Build history of the part. All positions in model axes, mm. A direction names the side the tool comes from. Round coordinates to 2 decimals unless told otherwise and drop trailing zeros. Order: outer loops, then holes, each group sorted by start corner. A loop starts at its lowest first (then second) coordinate and runs counter-clockwise, first axis right, second up. Notation, with made-up numbers: M 45,-6 L 70,-6 A13 ccw 70,7 Z; hole C -30.75,-6.5 d10. An arc over 180 degrees is marked long. Use CSV: the item, a comma, the result in double quotes.
Autodesk Inventor part; units mm, degrees
ref_plane "YZ Plane" through (0, 0, 0) normal (1, 0, 0) x (0, 1, 0)
ref_plane "XZ Plane" through (0, 0, 0) normal (0, 1, 0) x (-1, 0, 0)
ref_plane "XY Plane" through (0, 0, 0) normal (0, 0, 1) x (1, 0, 0)
sketch "Sketch1" plane through (0, 0, 0) normal (1, 0, 0) x (0, 1, 0)
  circle A0 centre (0, 0) radius 10
  circle A1 centre (0, 0) radius 20
  circle A2 centre (0, 0) radius 40
  circle A3 centre (0, 0) radius 50
  dimension "d0" = 20
  dimension "d1" = 40
  dimension "d2" = 80
  dimension "d3" = 100
extrude "Extrusion1" add sketch "Sketch1" along normal mid plane 40
extrude "Extrusion2" add sketch "Sketch1" along normal mid plane 30 contours A2
fillet "Fillet1" radius 2 1 edges at (-15, -40, 0)
fillet "Fillet4" radius 2 1 edges at (15, -40, 0)
fillet "Fillet5" radius 2 1 edges at (-15, -20, 0)
fillet "Fillet6" radius 2 1 edges at (15, -20, 0)
(1) Drop flat-ended pins along their axis: pin 1 (2 mm diameter, centred on y = 16.5, z = -15, fed in from -X); pin 2 (4 mm diameter, centred on y = -29.5, z = 23.5, fed in from +X); pin 3 (12 mm diameter, centred on x = 9, y = -35, fed in from -Z). Give the stop position or say it passes through.
Answer block:
pin 1,"stops at x = -15.13"
pin 2,"stops at x = 15.97"
pin 3,"stops at z = -40.73"
(2) Two-plate mould, pull along Y, no slides. Class faces 1 (the face through (18.479, -4.336, 19.524)), 2 (the face through (20, -5, 9)), 3 (the face through (-0.28, 47.69, -15.02)): released by +Y, released by -Y, zero draft, split by the parting line, or undercut.
Answer block:
face 1,"undercut"
face 2,"zero draft"
face 3,"split by the parting line"
(3) Tool access for faces 4 (the face through (-18.479, -4.336, -19.524)), 5 (the face through (15, 16, -16)), 6 (the face through (-0.28, -2.17, 9.76)): list every direction of +Z, -Z, +X, -X, +Y, -Y with a clear straight run to the whole face (end or side of a thin tool).
Answer block:
face 4,"-X"
face 5,"+X"
face 6,"+X, -X"
(4) Cut at C-C, the plane x = 3.5. Give the cut face in (y, z).
Answer block:
outline,"C 0,0 d100; hole C 0,0 d20"
(5) Cut at D-D, the plane z = -42. Give the cut face in (x, y).
Answer block:
outline,"M -20,-27.13 L 20,-27.13 L 20,27.13 L -20,27.13 Z"
(6) Wall check: line 1 (Z direction, x = -18.25, y = 0); line 2 (Z direction, x = 10, y = 0); line 3 (Z direction, x = 16, y = 7). Give the ranges that are in metal, low to high. Write a range as from..to.
Answer block:
line 1,"z = -50..-40, -20..-10, 10..20, 40..50"
line 2,"z = -50..-10, 10..50"
line 3,"z = -49.51..-39.11, -19.02..-7.14, 7.14..19.02, 39.11..49.51"
